```python
from build123d import *

# Parameters (mm, degrees)
F0_W     = 185
F0_H     = 110
F1_DEPTH = 5
F3_DEPTH = 10.001
F5_D     = 4.2
F5_DEPTH = 17.4
F5_TIP   = 1.2618073


with BuildPart() as f1:
    # F0 (on Front) → F1 (new body, symmetric)
    with BuildSketch(Plane.XZ):
        Rectangle(F0_W, F0_H)
    extrude(amount=F1_DEPTH, both=True)

    # F2 (on face) → F3 (cut, through all)
    with BuildSketch(Plane.XZ.offset(5)):
        with BuildLine():
            ThreePointArc((-63, 40), (-67.5, 44.5), (-72, 40))
            Line((-72, 40), (-72, 15))
            ThreePointArc((-72, 15), (-67.5, 10.5), (-63, 15))
            Line((-63, 15), (-63, 40))
        make_face()
        with BuildLine():
            ThreePointArc((-63, -15), (-67.5, -10.5), (-72, -15))
            Line((-72, -15), (-72, -40))
            ThreePointArc((-72, -40), (-67.5, -44.5), (-63, -40))
            Line((-63, -40), (-63, -15))
        make_face()
        with BuildLine():
            ThreePointArc((72, 40), (67.5, 44.5), (63, 40))
            Line((63, 40), (63, 15))
            ThreePointArc((63, 15), (67.5, 10.5), (72, 15))
            Line((72, 15), (72, 40))
        make_face()
        with BuildLine():
            ThreePointArc((72, -15), (67.5, -10.5), (63, -15))
            Line((63, -15), (63, -40))
            ThreePointArc((63, -40), (67.5, -44.5), (72, -40))
            Line((72, -40), (72, -15))
        make_face()
    extrude(amount=-F3_DEPTH, mode=Mode.SUBTRACT)

    # F5
    with Locations(Plane.XZ.offset(5)):
        with Locations((-17.5, 27.5), (-17.5, -12.5), (17.5, 27.5), (17.5, -12.5)):
            Hole(F5_D / 2, depth=F5_DEPTH)
            with Locations((0, 0, -(F5_DEPTH + F5_TIP / 2))):  # 118° drill point
                Cone(0, F5_D / 2, F5_TIP, mode=Mode.SUBTRACT)


solid = f1.part
```
Model file for the job. Use its own axes, mm. Round coordinates to 2 decimals unless told otherwise and drop trailing zeros. Order: outer loops, then holes, each group sorted by start corner. A loop starts at its lowest first (then second) coordinate and runs counter-clockwise, first axis right, second up. Notation, with made-up numbers: (46, -5.75) -> (59, -5.75) arc R7 cw to (59, 1.25) -> close; hole circle Ø4 at (27.5, -10). An arc over 180 degrees is marked (long way). Use one line per item in the form item = value.
Item 1: Flat gauge pin, fed straight in: pin 1 Ø5 at (x, z) = (17.5, -12.5) entering from -Y. Where does the tip first touch, or does it go through?
Returned:
pin_1 = -5
Item 2: Pull direction Z, two halves, no side cores. Call faces 1 (the face through (-1, 0, 55)), 2 (the face through (15.497, 0.07, -11.869)), 3 (the face through (-1, 0, -55)): released by +Z, released by -Z, zero draft, split by the parting line, or undercut.
Returned:
face_1 = released by +Z
face_2 = undercut
face_3 = released by -Z
Item 3: Cut at C-C, the plane z = -12.5. Write the cut outline in (x, y), and give its area (3 significant figures).
Returned:
outline = (-92.5, -5) -> (-71.24, -5) -> (-71.24, 5) -> (-92.5, 5) -> close; (-63.76, -5) -> (-19.6, -5) -> (-19.6, 5) -> (-63.76, 5) -> close; (-15.4, -5) -> (15.4, -5) -> (15.4, 5) -> (-15.4, 5) -> close; (19.6, -5) -> (63.76, -5) -> (63.76, 5) -> (19.6, 5) -> close; (71.24, -5) -> (92.5, -5) -> (92.5, 5) -> (71.24, 5) -> close
area = 1,620 mm^2
Item 4: Cut at A-A, the plane x = -67.5. Write the cut outline in (y, z).
Returned:
outline = (-5, -55) -> (5, -55) -> (5, -44.5) -> (-5, -44.5) -> close; (-5, -10.5) -> (5, -10.5) -> (5, 10.5) -> (-5, 10.5) -> close; (-5, 44.5) -> (5, 44.5) -> (5, 55) -> (-5, 55) -> close
Item 5: Cut at B-B, the plane y = -0.5. Give the number of separate pieces and of enclosed holes in the cut face, and give its area (3 significant figures).
Returned:
separate_pieces = 1
enclosed_holes = 8
area = 19,100 mm^2
Item 6: Drill centre lines: line 1 (Z direction, x = 17.5, y = 0); line 2 (X direction, y = 0.25, z = 33); line 3 (Z direction, x = -70, y = 4.25). Where is each one in solid material? Low to high.
Returned:
line_1 = -55 to -14.6, -10.4 to 25.4, 29.6 to 55
line_2 = -92.5 to -72, -63 to 63, 72 to 92.5
line_3 = -55 to -43.74, -11.26 to 11.26, 43.74 to 55
Item 7: Cut at D-D, the plane x = -17.5. Write the cut outline in (y, z), and give its area (3 significant figures).
Returned:
outline = (-5, -55) -> (5, -55) -> (5, -14.6) -> (-5, -14.6) -> close; (-5, -10.4) -> (5, -10.4) -> (5, 25.4) -> (-5, 25.4) -> close; (-5, 29.6) -> (5, 29.6) -> (5, 55) -> (-5, 55) -> close
area = 1,020 mm^2
